Could you check a few things on this drawing? It's one solid part, dimensions in mm from its lowest x, y, z. A direction names the side the tool comes from. Give positions to 0.01 mm unless a question says otherwise; leave off trailing zeros. Order: outer loops, then holes, each group sorted by start corner. A loop starts at its lowest first (then second) coordinate and runs counter-clockwise, first axis right, second up. Notation, with made-up numbers: M -38,6 L 10,6 A37 ccw 10,44 Z; hole C -4.5,-28 d2. An arc over 180 degrees is marked long. Use one line per item in the form item = value. Start each with the question number.
1. For the marked faces 4 and 5, which set-ups out of +Z, -Z, +X, -X, +Y, -Y let a thin tool reach every point of the face, with its end or its side?
2. Will this pin go through, and if not, where does the flat tip stop? P1, Ø6, axis at x = 65, z = 30, coming from the -Y side.
3. I need wall thicknesses on L1, parallel to Z at x = 21, y = 8.75 (1 decimal); L2, parallel to X at y = 5.5, z = 18; L3, parallel to Y at x = 62, z = 114.5. Which ranges of each line are inside material? Lowest first, please.
4. I want a section at D-D, the plane z = 70.5. List the corners of the cut face in (x, y) for me, and give its area (3 significant figures).
5. We'd pull the mould along Z, two halves only. Please class the marked faces 1, 2 and 3: +Z half, -Z half, draft (parallel to the pull), parting line (faces both ways), or undercut.
6. I want a section at C-C, the plane x = 51. List the corners of the cut face in (y, z) for me (1 decimal).
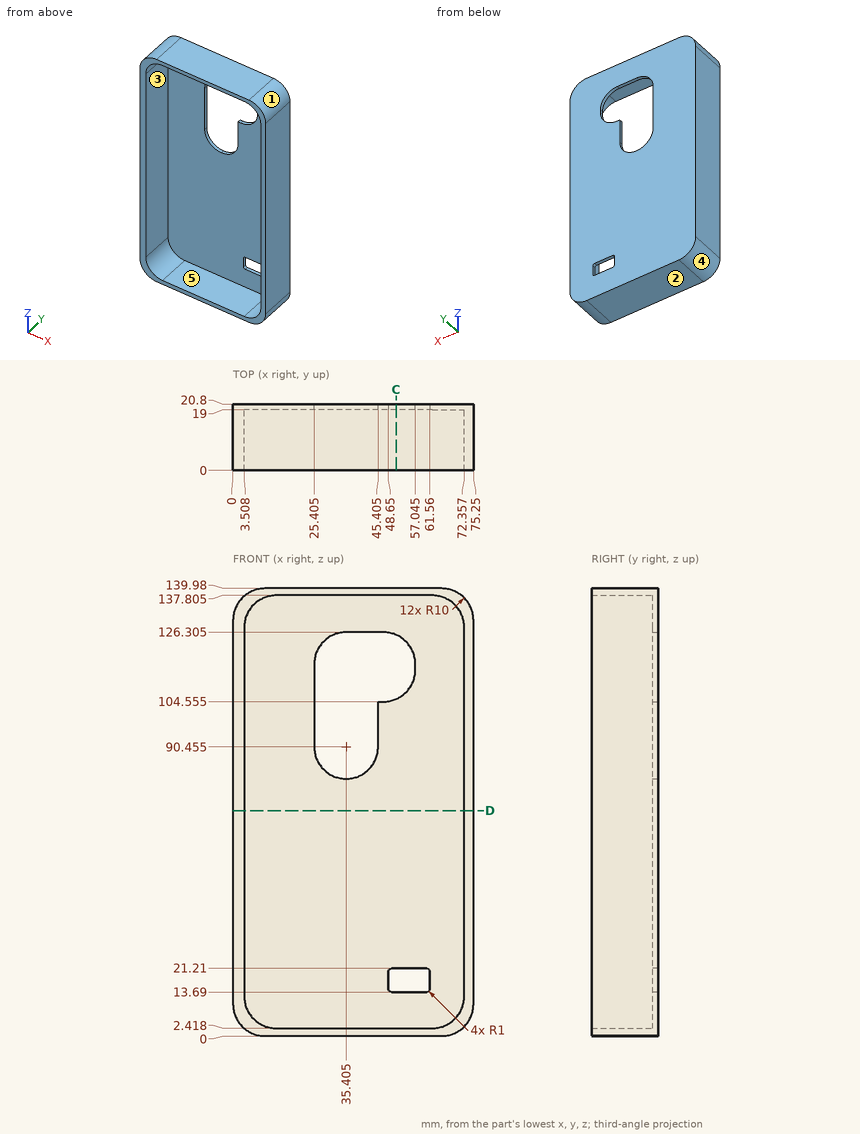
Check result:
q1.face_4 = -Z, -X, +Y, -Y
q1.face_5 = -Y
q2.P1 = 19
q3.L1 = 0 to 2.4, 137.8 to 140
q3.L2 = 0 to 3.51, 72.36 to 75.25
q3.L3 = 19 to 20.8
q4.outline = M 0,0 L 3.51,0 L 3.51,19 L 72.36,19 L 72.36,0 L 75.25,0 L 75.25,20.8 L 0,20.8 Z
q4.area = 257 mm2
q5.face_1 = +Z half
q5.face_2 = -Z half
q5.face_3 = undercut
q6.outline = M 0,0 L 20.8,0 L 20.8,13.7 L 19,13.7 L 19,2.4 L 0,2.4 Z; M 0,137.8 L 19,137.8 L 19,125.5 L 20.8,125.5 L 20.8,140 L 0,140 Z; M 19,21.2 L 20.8,21.2 L 20.8,105.4 L 19,105.4 Z
